Can you work these out from the model? Positions are in its coordinate system, mm. Face numbers are marked on the shaded views. A direction names the side the tool comes from. Give positions to 0.01 mm unless a question says otherwise; leave off trailing zeros. Loops run counter-clockwise (first coordinate to the right, second up) from the corner with the lowest first, then second, coordinate; pieces in that order, holes last. Notation, with made-up numbers: (41.25, 62) - (68.25, 62) arc R26 ccw to (68.25, 84) - close; hole circle Ø1 at (56.25, -18.5). An arc over 180 degrees is marked (long way). Use a Markdown table: item, result. Add a question column.
```python
from build123d import *

# Parameters (mm, degrees)
EXTRUDE_1_DEPTH     = 50
SKETCH_5_R          = 4.5
CUT_EXTRUDE_1_DEPTH = 97
SKETCH_6_R          = 2.5
CUT_EXTRUDE_2_DEPTH = 97
SKETCH_7_R          = 2.5
CUT_EXTRUDE_3_DEPTH = 97


with BuildPart() as part:
    # 스케치4 → 보스-돌출1 (new body)
    with BuildSketch(Plane.XY):
        Polygon((40, 0), (0, 0), (-40, 0), (-40, 10), (-30, 10), (-30, 40), (30, 40), (30, 10), (40, 10), align=None)
    extrude(amount=EXTRUDE_1_DEPTH)

    # 스케치5 → 컷-돌출1 (cut)
    with BuildSketch(Plane.XY.offset(50)):
        with Locations((0, 25)):
            Circle(SKETCH_5_R)
        Polygon((0, 25), (15, 40), (-15, 40), align=None)
    extrude(amount=-CUT_EXTRUDE_1_DEPTH, mode=Mode.SUBTRACT)

    # 스케치6 → 컷-돌출2 (cut)
    with BuildSketch(Plane(origin=(0, 10, 0), x_dir=(1, 0, 0), z_dir=(0, 1, 0))):
        with Locations((-35, -10)):
            Circle(SKETCH_6_R)
        with Locations((-35, -40)):
            Circle(SKETCH_6_R)
    extrude(amount=-CUT_EXTRUDE_2_DEPTH, mode=Mode.SUBTRACT)

    # 스케치7 → 컷-돌출3 (cut)
    with BuildSketch(Plane(origin=(0, 10, 0), x_dir=(1, 0, 0), z_dir=(0, 1, 0))):
        with Locations((35, -10)):
            Circle(SKETCH_7_R)
        with Locations((35, -40)):
            Circle(SKETCH_7_R)
    extrude(amount=-CUT_EXTRUDE_3_DEPTH, mode=Mode.SUBTRACT)


solid = part.part
```
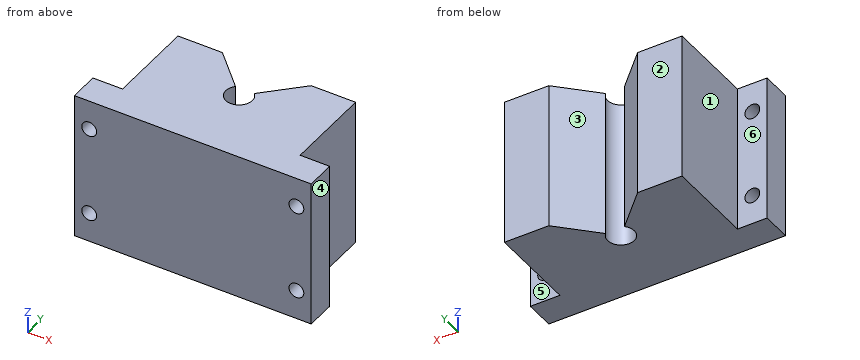
1. Suppose I cut it at B-B (z = 40). List the corners of the cut face in (x, y) for me.
2. Please list where these lines run through material, in increasing order: line 1 along X through (y, z) = (7, 10); line 2 along Z through (x, y) = (35, 2); line 3 along Z through (x, y) = (-36, 3). Write a range as [from, to].
3. Suppose I cut it at D-D (y = 8.5). List the corners of the cut face in (x, z) for me.
4. On a 3-axis mill with a long thin cutter (end or side, diameter ignored), from which of +Z, -Z, +X, -X, +Y, -Y can I reach the whole of each face in a straight line? I mean the marked faces 4, 5 and 6. Say none if no direction works.
5. Will these pins go through, and if not, where does the flat tip stop? P1, Ø3, axis at x = 34, z = 17.5, coming from the +Y side; P2, Ø2, axis at x = 13.5, z = 31, coming from the -Y side; P3, Ø9, axis at y = 32, z = 30, coming from the -X side; P4, Ø4.5, axis at x = -35, z = 10, coming from the -Y side.
6. Suppose I cut it at C-C (y = 25). List the corners of the cut face in (x, z) for me.
7. If we mould it in two halves opening along X, with no side actions, what happens to the marked faces 1, 2 and 3? For each: released by +X, released by -X, zero draft, split by the parting line, or undercut.
8. Suppose I cut it at A-A (x = -35). List the corners of the cut face in (y, z) for me, and give its area (3 significant figures).
Results below:
| question | item | result |
|---|---|---|
| 1 | outline | (-40, 0) - (-37.5, 0) - (-37.5, 10) - (-40, 10) - close; (-32.5, 0) - (32.5, 0) - (32.5, 10) - (30, 10) - (30, 40) - (15, 40) - (3.18, 28.18) arc R4.5 cw (long way) to (-3.18, 28.18) - (-15, 40) - (-30, 40) - (-30, 10) - (-32.5, 10) - close; (37.5, 0) - (40, 0) - (40, 10) - (37.5, 10) - close |
| 2 | line 1 | [-40, -37.5], [-32.5, 32.5], [37.5, 40] |
| 2 | line 2 | [0, 7.5], [12.5, 37.5], [42.5, 50] |
| 2 | line 3 | [0, 7.71], [12.29, 37.71], [42.29, 50] |
| 3 | outline | (-40, 0) - (40, 0) - (40, 50) - (-40, 50) - close; hole circle Ø5 at (-35, 10); hole circle Ø5 at (-35, 40); hole circle Ø5 at (35, 10); hole circle Ø5 at (35, 40) |
| 4 | face 4 | +Z, -Z, +X, +Y, -Y |
| 4 | face 5 | +Z, -Z, +X, +Y |
| 4 | face 6 | +Z, -Z, -X, +Y |
| 5 | P1 | y = 10 |
| 5 | P2 | y = 0 |
| 5 | P3 | x = -30 |
| 5 | P4 | through |
| 6 | outline | (-30, 0) - (-4.5, 0) - (-4.5, 50) - (-30, 50) - close; (4.5, 0) - (30, 0) - (30, 50) - (4.5, 50) - close |
| 7 | face 1 | released by -X |
| 7 | face 2 | zero draft |
| 7 | face 3 | undercut |
| 8 | outline | (0, 0) - (10, 0) - (10, 7.5) - (0, 7.5) - close; (0, 12.5) - (10, 12.5) - (10, 37.5) - (0, 37.5) - close; (0, 42.5) - (10, 42.5) - (10, 50) - (0, 50) - close |
| 8 | area | 400 mm² |
